Autodesk Inventor part; units mm, degrees
ref_plane "YZ Plane" through (0, 0, 0) normal (1, 0, 0) x (0, 1, 0)
ref_plane "XZ Plane" through (0, 0, 0) normal (0, 1, 0) x (-1, 0, 0)
ref_plane "XY Plane" through (0, 0, 0) normal (0, 0, 1) x (1, 0, 0)
sketch "Sketch1" plane through (0, 0, 0) normal (1, 0, 0) x (0, 1, 0)
  line L0 (-75, 25) -> (75, 25)
  line L1 (75, 25) -> (75, -25)
  line L2 (75, -25) -> (-75, -25)
  line L3 (-75, -25) -> (-75, 25)
  point P0 (0, 0)
  dimension "d0" = 150
  dimension "d1" = 50
  dimension "d2" = 25
  dimension "d3" = 75
extrude "Extrusion1" add sketch "Sketch1" along normal blind 6
sketch "Sketch2" plane through (6, 0, 0) normal (1, 0, 0) x (0, 0, -1)
  point P0 (0, 0)
  point P1 (0, 0)
  point P2 (0, 50)
  point P3 (0, -50)
  dimension "d15" = 50
  dimension "d16" = 50
hole "Hole2" at (6, 0, 0) at (6, 50, 0) at (6, -50, 0) direction (-1, 0, 0) diameter 12 end through all
fillet "Fillet3" radius 12 2 edges at (3, 75, 25) (3, 75, -25)
equation "\"d0\" = 3 * hoop_tabs_width"
equation "\"d1\" = hoop_tabs_width"
equation "\"d4\" = hoop_tabs_thickness"
equation "\"d17\" = hoop_tabs_hole"
equation "\"d24\" = hoop_tabs_hole"
equation "\"hoop_tabs_width\" = 50"
equation "\"hoop_tabs_thickness\" = 6"
equation "\"hoop_tabs_hole\" = 12"
equation "\"hoop_angle_z\" = 45deg"
equation "\"hoop_bearing_length\" = 5deg"
equation "\"hoop_cable_diam\" = 5"
equation "\"hoop_cable_pulley_diam\" = 22"
equation "\"hoop_thickness_large\" = 4"
equation "\"hoop_thickness_medium\" = 3.2"
equation "\"hoop_thickness_small\" = 2"
equation "\"hoop_width_large\" = 51"
equation "\"hoop_width_medium\" = 33.7"
equation "\"hoop_width_small\" = 25.4"
equation "\"rack_tooth_addendum\" = 5"
equation "\"rack_tooth_dedendum\" = 5"
equation "\"rack_tooth_thickness\" = 5"
equation "\"secure_arm_angle\" = 35deg"
equation "\"secure_arm_radii\" = 9"
equation "\"support_baseClamp_platformLengthBuffer\" = 35"
equation "\"support_baseClamp_platformThickness\" = 15"
equation "\"support_baseClamp_platformWidthBuffer\" = 0"
equation "\"support_baseClamp_sleeveHoleDiameter\" = 12"
equation "\"support_baseClamp_sleeveSweepTerminationAngle\" = 55deg"
equation "\"support_baseClamp_thickness\" = 8"
equation "\"support_frame_endHoleBuffer\" = 45"
equation "\"support_frame_squareBarFillet\" = 2"
equation "\"support_frame_squareBarThickness\" = 5"
equation "\"wheelchair_deployed_width\" = 635"
equation "\"wheelchair_deployed_length\" = 1067"
equation "\"wheelchair_deployed_height\" = 914"
equation "\"sm_varx_squareBarThickness\" = 2.5"
equation "\"sm_varx_pinPlate_thickness\" = 5"
equation "\"sm_varx_pinPlate_holeDiameter\" = 5"
equation "\"sm_varx_member_tolerance\" = 0"
equation "\"hoop_bushing23_radialInterference\" = 0"
equation "\"hoop_bushing12_radialInterference\" = 0"
equation "\"hoop_bushing23_od\" = -2 * hoop_thickness_medium + hoop_width_medium + hoop_bushing23_radialInterference"
equation "\"hoop_bushing12_od\" = -2 * hoop_thickness_large + hoop_width_large + hoop_bushing12_radialInterference"
equation "\"wheelchatir_pos_deploy_angle_0\" = 65deg"
equation "\"wheelchatir_pos_store_angle_0\" = 90deg"
equation "\"wheelchatir_pos_deploy_angle_1\" = 20deg"
equation "\"wheelchatir_pos_store_angle_1\" = 20deg"
equation "\"hoop_bushing12_thickness\" = -hoop_width_medium + hoop_bushing12_od - 2 * hoop_bushing12_radialInterference"
equation "\"hoop_bushing23_thickness\" = -hoop_width_small + hoop_bushing23_od - 2 * hoop_bushing23_radialInterference"
properties part number "hoop_tab" material "Steel, Mild"
The model under review builds one solid part; all positions refer to its coordinate system, in mm. Round coordinates to 2 decimals unless told otherwise and drop trailing zeros. Order: outer loops, then holes, each group sorted by start corner. A loop starts at its lowest first (then second) coordinate and runs counter-clockwise, first axis right, second up. Notation, with made-up numbers: (13.5, 80) -> (52.5, 80) arc R27 ccw to (52.5, 114) -> close; hole circle Ø6 at (7.25, -2). An arc over 180 degrees is marked (long way). Write item = value, one per line. Start each with the question number.
Item 1: Consider section D-D on y = -52. Write out the cut boundary in (x, z).
Item 2: Consider section B-B on z = 0. Write out the cut boundary in (x, y).
Item 3: For line 1 along Y through (x, z) = (3.7, 0); line 2 along Y through (x, z) = (4.65, -1); line 3 along Z through (x, y) = (3.9, -50), list the stretches that pass through material, from the lowest coordinate up.
Item 4: Consider section C-C on x = 4.65. Write out the cut boundary in (y, z).
Item 5: Consider section A-A on y = 50. Write out the cut boundary in (x, z).
Item 6: Mouldability with a two-part tool opening along Y and no side actions: class faces 1 (the face through (3, 75, 0)), 2 (the face through (3, -7, 25)), 3 (the face through (3, -75, 0)), 4 (the face through (2.958, -44.143, 1.301)) as released by +Y, released by -Y, zero draft, split by the parting line, or undercut.
Conclusion:
q1.outline = (0, -25) -> (6, -25) -> (6, -5.66) -> (0, -5.66) -> close; (0, 5.66) -> (6, 5.66) -> (6, 25) -> (0, 25) -> close
q2.outline = (0, -75) -> (6, -75) -> (6, -56) -> (0, -56) -> close; (0, -44) -> (6, -44) -> (6, -6) -> (0, -6) -> close; (0, 6) -> (6, 6) -> (6, 44) -> (0, 44) -> close; (0, 56) -> (6, 56) -> (6, 75) -> (0, 75) -> close
q3.line_1 = -75 to -56, -44 to -6, 6 to 44, 56 to 75
q3.line_2 = -75 to -55.92, -44.08 to -5.92, 5.92 to 44.08, 55.92 to 75
q3.line_3 = -25 to -6, 6 to 25
q4.outline = (-75, -25) -> (63, -25) arc R12 ccw to (75, -13) -> (75, 13) arc R12 ccw to (63, 25) -> (-75, 25) -> close; hole circle Ø12 at (-50, 0); hole circle Ø12 at (0, 0); hole circle Ø12 at (50, 0)
q5.outline = (0, -25) -> (6, -25) -> (6, -6) -> (0, -6) -> close; (0, 6) -> (6, 6) -> (6, 25) -> (0, 25) -> close
q6.face_1 = released by +Y
q6.face_2 = zero draft
q6.face_3 = released by -Y
q6.face_4 = undercut
